Geometry: final body of the model. Coordinates: model frame, mm. Coordinates: 2 decimals unless noted, no trailing zeros. Write each loop counter-clockwise with the first axis right and the second up, starting at its lowest first coordinate (ties: lowest second). Pieces come first, ordered by that corner, then holes. Notation, with made-up numbers: M 66,74.5 L 78,74.5 A25 cw 78,110.5 Z; hole C 6.5,-5 d5. An arc over 180 degrees is marked long. Write item = value, one per line. Start each with the question number.
Item 1: Section C-C on z = 56. Output: boundary loops of the cut face in (x, y).
Item 2: Section A-A on x = 0. Output: boundary loops of the cut face in (y, z), plus the area to 3 significant figures.
Item 3: Ray query, L1, parallel to Z at x = -3, y = -4; L2, parallel to X at y = 0, z = 42. Return the intervals inside material, ascending. Write a range as [from, to].
Item 4: First-contact query: pin 1 Ø4 at (y, z) = (-2, 50.5) entering from -X; pin 2 Ø1 at (x, y) = (-4, -1) entering from +Z; pin 3 Ø2 at (x, z) = (3.5, 32.5) entering from -Y; pin 4 Ø5 at (x, z) = (0.5, 33) entering from -Y. Flat tips, straight axial feed; report the tip coordinate or a pass-through.
Item 5: Section D-D on y = -4. Output: boundary loops of the cut face in (x, z).
from build123d import *

# Parameters (mm, degrees)
SKETCH1_R           = 6
BOSS_EXTRUDE1_DEPTH = 4
SKETCH2_R           = 2
BOSS_EXTRUDE2_DEPTH = 85
SKETCH3_R           = 0.25


with BuildPart() as part:
    # Sketch1 → Boss-Extrude1 (new body)
    with BuildSketch(Plane.XY):
        Circle(SKETCH1_R)
    extrude(amount=BOSS_EXTRUDE1_DEPTH)

    # Sketch2 → Boss-Extrude2 (add)
    with BuildSketch(Plane.XY):
        Circle(SKETCH2_R)
    extrude(amount=BOSS_EXTRUDE2_DEPTH)

    # Sketch3 → Cut-Revolve1 (revolve, cut)
    with BuildSketch(Plane(origin=(0, 0, 0), x_dir=(0, 0, -1), z_dir=(1, 0, 0))):
        with Locations((-74, 2)):
            Circle(SKETCH3_R)
    revolve(axis=Axis((0, 0, 0), (0, 0, 1)), mode=Mode.SUBTRACT)


solid = part.part
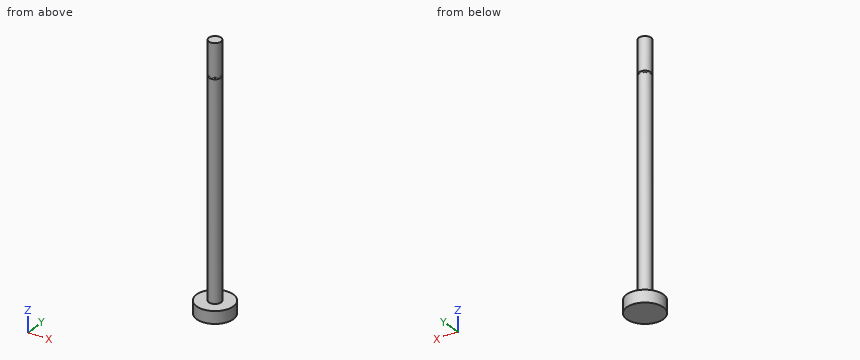
Responses:
q1.outline = C 0,0 d4
q2.outline = M -6,0 L 6,0 L 6,4 L 2,4 L 2,73.75 A0.25 cw 2,74.25 L 2,85 L -2,85 L -2,74.25 A0.25 cw -2,73.75 L -2,4 L -6,4 Z
q2.area = 372 mm²
q3.L1 = [0, 4]
q3.L2 = [-2, 2]
q4.pin_1 = -2
q4.pin_2 = 4
q4.pin_3 = through
q4.pin_4 = -2
q5.outline = M -4.47,0 L 4.47,0 L 4.47,4 L -4.47,4 Z
